Here's how the part is built. I have some questions about the finished solid (model axes, mm). Face numbers are marked on the shaded views. A direction names the side the tool comes from. Round coordinates to 2 decimals unless told otherwise and drop trailing zeros. Order: outer loops, then holes, each group sorted by start corner. A loop starts at its lowest first (then second) coordinate and runs counter-clockwise, first axis right, second up. Notation, with made-up numbers: (47.5, 3) - (72.5, 3) arc R25 ccw to (72.5, 38) - close; hole circle Ø4 at (15, 64). An arc over 180 degrees is marked (long way). Answer as a JSON object with one key per item and string values.
```python
from build123d import *

# Parameters (mm, degrees)
SKETCH1_R           = 5.0038
BOSS_EXTRUDE1_DEPTH = 1.6002
SKETCH2_R           = 2.38125
BOSS_EXTRUDE2_DEPTH = 20.955
FILLET1_R           = 2.54


with BuildPart() as part:
    # Sketch1 → Boss-Extrude1 (new body)
    with BuildSketch(Plane.XY):
        Circle(SKETCH1_R)
    extrude(amount=BOSS_EXTRUDE1_DEPTH)

    # Sketch2 → Boss-Extrude2 (add)
    with BuildSketch(Plane.XY):
        Circle(SKETCH2_R)
    extrude(amount=-BOSS_EXTRUDE2_DEPTH)

    # Fillet1
    # the kernel refuses this fillet: 2.54 mm, written as the material it takes off along each edge
    with BuildSketch(Plane(origin=(0, 0, 1.6002), x_dir=(1, 0, 0), z_dir=(0, -1, 0))) as fillet1_piece_1:
        with BuildLine():
            CenterArc((2.644059345, -2.54), FILLET1_R, 21.715617283, 68.284382717)
            Line((2.644059345, 0), (2.644059345, 0.0508))
            Line((2.644059345, 0.0508), (5.0038, 0.0508))
            Line((5.0038, 0.0508), (5.0546, 0))
            ThreePointArc((5.0546, 0), (5.0546, -0.8001), (5.050994813, -1.581404))
            Line((5.050994813, -1.581404), (5.0038, -1.6002))
        make_face()
    revolve(axis=Axis((0, 0, 1.6002), (0, 0, 1)), mode=Mode.SUBTRACT)


solid = part.part
```
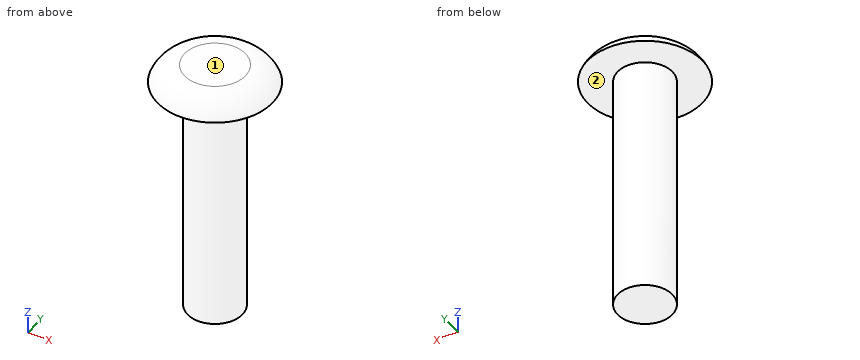
1. For P1, Ø1, axis at x = 3.5, y = 0, coming from the +Z side; P2, Ø1.5, axis at x = 1, y = 3, coming from the -Z side; P3, Ø1, axis at y = 4, z = -2.5, coming from the -X side (3 decimals); P4, Ø4, axis at x = 0, z = -11, coming from the +Y side, each with a flat end and sliding along its axis, tell me the tip position at first contact or that it passes through.
Responses:
{"P1": "z = 1.58", "P2": "z = 0", "P3": "through", "P4": "y = 2.38"}
2. If I drill on L1, parallel to Z at x = -2, y = -1.75; L2, parallel to X at y = 1.5, z = -2.75; L3, parallel to Z at x = 1.5, y = 3.75, over which ranges is the centre line in solid material (lowest first)? Write a range as [from, to].
Responses:
{"L1": "[0, 1.6]", "L2": "[-1.85, 1.85]", "L3": "[0, 1.18]"}
3. For the marked faces 1 and 2, which set-ups out of +Z, -Z, +X, -X, +Y, -Y let a thin tool reach every point of the face, with its end or its side?
Responses:
{"face 1": "+Z, +X, -X, +Y, -Y", "face 2": "-Z"}
4. Imagine slicing it at C-C (z = -14.75). List the corners of the cut face in (x, y) for me, plus the area to 3 significant figures.
Responses:
{"outline": "circle Ø4.76 at (0, 0)", "area": "17.8 mm2"}
5. Imagine slicing it at A-A (y = 0). List the corners of the cut face in (x, z) for me (3 decimals).
Responses:
{"outline": "(-5.004, 0) - (-2.381, 0) - (-2.381, -20.955) - (2.381, -20.955) - (2.381, 0) - (5.004, 0) arc R2.54 ccw to (2.644, 1.6) - (-2.644, 1.6) arc R2.54 ccw to start"}
